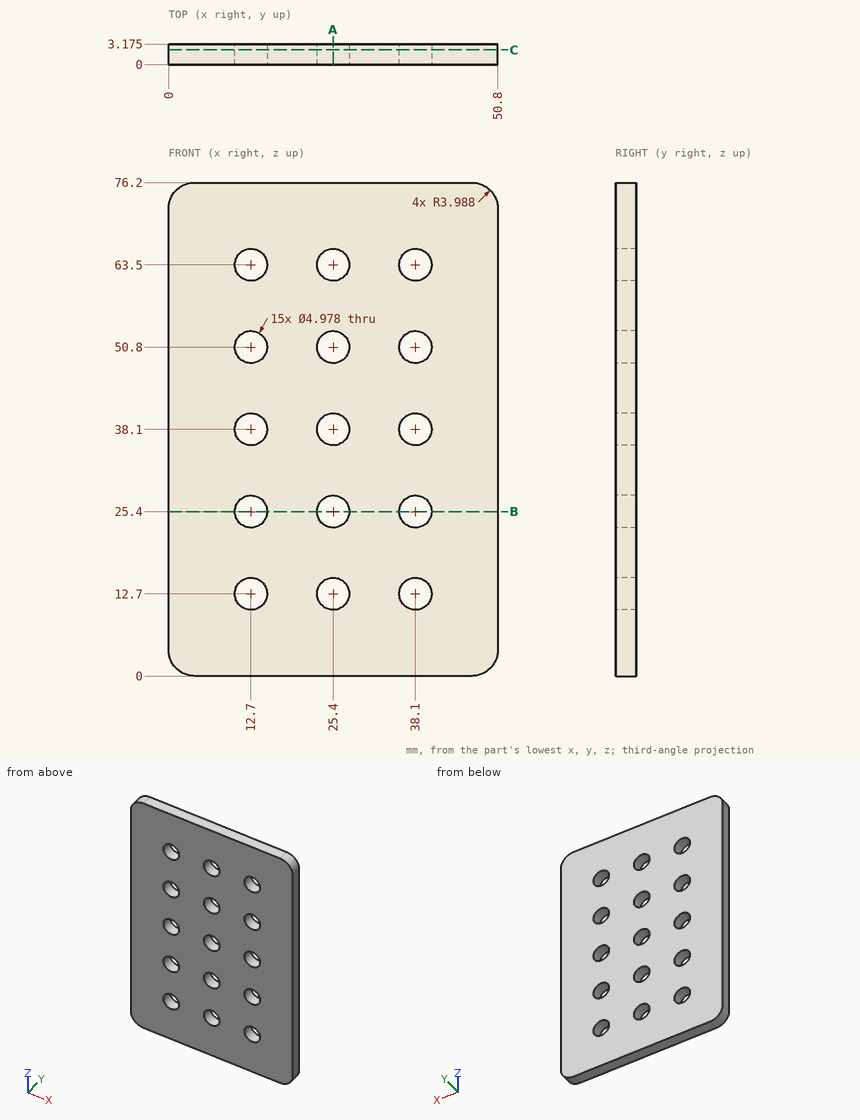
For this review, use the dimensioned drawing (mm, ordinates from the lowest corner) and the shaded views. Coordinates: 2 decimals unless noted, no trailing zeros. Write each loop counter-clockwise with the first axis right and the second up, starting at its lowest first coordinate (ties: lowest second). Pieces come first, ordered by that corner, then holes. Notation, with made-up numbers: (77.5, 88) - (112.5, 88) arc R9 ccw to (112.5, 103) - close; hole circle Ø10 at (-15.5, 68). An arc over 180 degrees is marked (long way). Answer in a Markdown table with one row per item. Add a question column.
Q1. Consider section B-B on z = 25.4. Give the boundary of the cut face in (x, y) (1 decimal), then the cut area to 3 significant figures.
Q2. Consider section C-C on y = 2.25. Give the number of separate pieces and of enclosed holes in the cut face.
Q3. Consider section A-A on x = 25.4. Give the boundary of the cut face in (y, z) (1 decimal), then the cut area to 3 significant figures.
Q4. To check wall thickness, follow line 1 along Z through (x, y) = (25.4, 1); line 2 along X through (y, z) = (0.2, 53) (1 decimal); line 3 along Z through (x, y) = (24, 1). State the ranges of each line that lie inside material, in increasing order. Write a range as from..to.
Q5. Clearance check with a flat-ended pin moving along its axis: pin 1 (1.5 mm diameter, centred on y = 2, z = 7.5, fed in from -X). State where the tip first meets the part, or that it passes through.
Answers below:
| question | item | result |
|---|---|---|
| 1 | outline | (0, 0) - (10.2, 0) - (10.2, 3.2) - (0, 3.2) - close; (15.2, 0) - (22.9, 0) - (22.9, 3.2) - (15.2, 3.2) - close; (27.9, 0) - (35.6, 0) - (35.6, 3.2) - (27.9, 3.2) - close; (40.6, 0) - (50.8, 0) - (50.8, 3.2) - (40.6, 3.2) - close |
| 1 | area | 114 mm² |
| 2 | separate pieces | 1 |
| 2 | enclosed holes | 15 |
| 3 | outline | (0, 0) - (3.2, 0) - (3.2, 10.2) - (0, 10.2) - close; (0, 15.2) - (3.2, 15.2) - (3.2, 22.9) - (0, 22.9) - close; (0, 27.9) - (3.2, 27.9) - (3.2, 35.6) - (0, 35.6) - close; (0, 40.6) - (3.2, 40.6) - (3.2, 48.3) - (0, 48.3) - close; (0, 53.3) - (3.2, 53.3) - (3.2, 61) - (0, 61) - close; (0, 66) - (3.2, 66) - (3.2, 76.2) - (0, 76.2) - close |
| 3 | area | 163 mm² |
| 4 | line 1 | 0..10.21, 15.19..22.91, 27.89..35.61, 40.59..48.31, 53.29..61.01, 65.99..76.2 |
| 4 | line 2 | 0..11.5, 13.9..24.2, 26.6..36.9, 39.3..50.8 |
| 4 | line 3 | 0..10.64, 14.76..23.34, 27.46..36.04, 40.16..48.74, 52.86..61.44, 65.56..76.2 |
| 5 | pin 1 | x = 0 |
